Geometry check sheet. Reference: the model listing, model coordinates, mm. Face numbers are marked on the shaded views. Coordinates: 2 decimals unless noted, no trailing zeros. Write each loop counter-clockwise with the first axis right and the second up, starting at its lowest first coordinate (ties: lowest second). Pieces come first, ordered by that corner, then holes. Notation, with made-up numbers: M 50.25,39 L 87.25,39 A14 ccw 87.25,61 Z; hole C -28,37.25 d1. An arc over 180 degrees is marked long. Write each question's results on one line, items separated by ' | '.
```python
from build123d import *

# Parameters (mm, degrees)
SKETCH_1_W          = 64
SKETCH_1_H          = 18
SKETCH_1_R          = 3
EXTRUDE_1_DEPTH     = 5
SKETCH_2_R          = 5.5
CUT_EXTRUDE_1_DEPTH = 3


with BuildPart() as part:
    # Sketch 1 → Extrude 1 (new body)
    with BuildSketch(Plane.XY):
        with Locations((3.920861217, 0.862610936)):
            Rectangle(SKETCH_1_W, SKETCH_1_H)
        with Locations((-11.079138783, 0.862610936)):
            Circle(SKETCH_1_R, mode=Mode.SUBTRACT)
        with Locations((18.920861217, 0.862610936)):
            Circle(SKETCH_1_R, mode=Mode.SUBTRACT)
    extrude(amount=EXTRUDE_1_DEPTH)

    # Sketch 2 → Cut-Extrude 1 (cut)
    with BuildSketch(Plane.XY.offset(5)):
        with Locations((-11.079138783, 0.862610936)):
            Circle(SKETCH_2_R)
        with Locations((18.920861217, 0.862610936)):
            Circle(SKETCH_2_R)
    extrude(amount=-CUT_EXTRUDE_1_DEPTH, mode=Mode.SUBTRACT)

    # Sketch 5 → Cut-Revolve 1 (revolve, cut)
    with BuildSketch(Plane(origin=(0, 0.862610936, 0), x_dir=(1, 0, 0), z_dir=(0, 1, 0)), mode=Mode.PRIVATE) as cut_revolve_1_sk:
        Polygon((-11.079138783, -5), (-16.079138783, -5), (-15.079138783, 0), (-11.079138783, 0), align=None)
    revolve(cut_revolve_1_sk.sketch.rotate(Axis((-11.079138783, 0.862610936, 0), (0, 0, 1)), 180), axis=Axis((-11.079138783, 0.862610936, 0), (0, 0, 1)), mode=Mode.SUBTRACT)

    # Sketch 5_4 → Cut-Revolve 2 (revolve, cut)
    with BuildSketch(Plane(origin=(0, 0.862610936, 0), x_dir=(1, 0, 0), z_dir=(0, 1, 0))):
        Polygon((18.920999606, -5), (23.920999606, -5), (22.920999606, 0), (18.920999606, 0), align=None)
    revolve(axis=Axis((18.920999606, 0.862610936, 0), (0, 0, 1)), mode=Mode.SUBTRACT)


solid = part.part
```
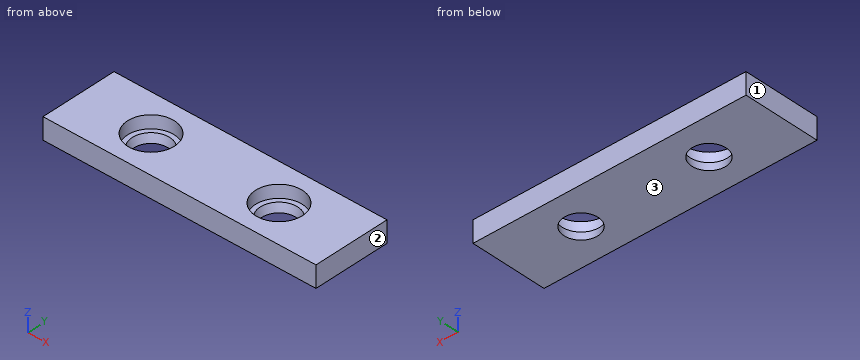
Q1. Sectioned sample at A-A on z = 4.25. Record the cut outline in (x, y), and give its area (3 significant figures).
Geometry check:
outline: M -28.08,-8.14 L 35.92,-8.14 L 35.92,9.86 L -28.08,9.86 Z; hole C -11.08,0.86 d11; hole C 18.92,0.86 d11 | area: 962 mm2
Q2. Mould release check, pull along X, two halves, no side actions. Record for the marked faces 1, 2 and 3: pulls with the +X half, pulls with the -X half, needs draft (parallel to the pull), parting line crosses it, or undercut.
Geometry check:
face 1: pulls with the -X half | face 2: pulls with the +X half | face 3: needs draft
Q3. Scan lines: probe 1 along X at (y, z) = (-2.25, 3.05); probe 2 along X at (y, z) = (3.75, 4.45); probe 3 along Y at (x, z) = (22.5, 3.05). Record each from-to range of solid material in increasing order.
Geometry check:
probe 1: x = -28.08 to -15.61, -6.54 to 14.39, 23.46 to 35.92 | probe 2: x = -28.08 to -15.76, -6.4 to 14.24, 23.6 to 35.92 | probe 3: y = -8.14 to -3.31, 5.04 to 9.86
Q4. Sectioned sample at C-C on z = 1.15. Record the cut outline in (x, y), and give its area (3 significant figures).
Geometry check:
outline: M -28.08,-8.14 L 35.92,-8.14 L 35.92,9.86 L -28.08,9.86 Z; hole C -11.08,0.86 d8.46; hole C 18.92,0.86 d8.46 | area: 1,040 mm2
Q5. Sectioned sample at B-B on y = -2.25. Give the number of separate pieces and of enclosed holes in the cut face, and give its area (3 significant figures).
Geometry check:
separate pieces: 3 | enclosed holes: 0 | area: 243 mm2
Q6. Depth check by flat-ended pin: P1, Ø9, axis at x = -11.08, y = 0.86, coming from the +Z side; P2, Ø9, axis at x = -9.5, y = 0.5, coming from the +Z side. Enter the tip coordinate at first touch or a pass-through.
Geometry check:
P1: stops at z = 2 | P2: stops at z = 5
